```python
from build123d import *

# Parameters (mm, degrees)
SKETCH1_R           = 5
SKETCH1_R_2         = 1.5
BOSS_EXTRUDE1_DEPTH = 5
BOSS_EXTRUDE4_DEPTH = 10
FILLET5_R           = 3
FILLET7_R           = 8
CUT_EXTRUDE6_DEPTH  = 10
FILLET9_R           = 1
FILLET11_R          = 0.1


with BuildPart() as part:
    # Sketch1 → Boss-Extrude1 (new, symmetric)
    # profile 1 of 3: a face of its own
    with BuildSketch(Plane(origin=(0, 0, 0), x_dir=(0, 0, -1), z_dir=(1, 0, 0))):
        with BuildLine():
            ThreePointArc((-11, 0), (-12.464466094, -3.535533906), (-16, -5))
            Line((-16, -5), (16, -5))
            ThreePointArc((16, -5), (11, 0), (16, 5))
            Line((16, 5), (-16, 5))
            ThreePointArc((-16, 5), (-12.464466094, 3.535533906), (-11, 0))
        make_face()
    # profile 2 of 3: a face of its own
    with BuildSketch(Plane(origin=(0, 0, 0), x_dir=(0, 0, -1), z_dir=(1, 0, 0))):
        with Locations((-16, 0)):
            Circle(SKETCH1_R)
        with Locations((-16, 0)):
            Circle(SKETCH1_R_2, mode=Mode.SUBTRACT)
    # profile 3 of 3: a face of its own
    with BuildSketch(Plane(origin=(0, 0, 0), x_dir=(0, 0, -1), z_dir=(1, 0, 0))):
        with Locations((16, 0)):
            Circle(SKETCH1_R)
        with Locations((16, 0)):
            Circle(SKETCH1_R_2, mode=Mode.SUBTRACT)
    extrude(amount=BOSS_EXTRUDE1_DEPTH, both=True)

    # Sketch6 → Boss-Extrude4 (add)
    with BuildSketch(Plane(origin=(5, 0, 0), x_dir=(0, 0, -1), z_dir=(1, 0, 0))):
        with BuildLine():
            Line((20.375428035, -2.419840804), (37.626356882, 0))
            Line((37.626356882, 0), (37.626356882, -5.863506349))
            Line((37.626356882, -5.863506349), (56, -2.931753174))
            Line((56, -2.931753174), (56, -0.788607304))
            Line((56, -0.788607304), (56, 5))
            Line((56, 5), (16, 5))
            ThreePointArc((16, 5), (20.30692489, 2.539763373), (20.375428035, -2.419840804))
        make_face()
    extrude(amount=-BOSS_EXTRUDE4_DEPTH)

    # Fillet5
    fillet5_edges = [part.edges().sort_by_distance(p)[0] for p in [
        (0, 0, -37.626356882),
    ]]
    fillet(fillet5_edges, radius=FILLET5_R)

    # Fillet7
    # the kernel refuses this fillet: 8 mm, written as the material it takes off along each edge
    with BuildSketch(Plane(origin=(25, 5, -56), x_dir=(0, -1, 0), z_dir=(-1, 0, 0))) as fillet7_piece_1:
        with BuildLine():
            CenterArc((FILLET7_R, FILLET7_R), FILLET7_R, 180, 90)
            Line((0, FILLET7_R), (0, 0))
            Line((0, 0), (FILLET7_R, 0))
        make_face()
    extrude(amount=50, mode=Mode.SUBTRACT)

    # Sketch8 → Cut-Extrude6 (cut)
    with BuildSketch(Plane(origin=(5, 0, 0), x_dir=(0, 0, -1), z_dir=(1, 0, 0))):
        Polygon((56, -2.931753174), (55.020132037, -1.951885211), (54.570397118, -3.159864865), (54.024984262, -3.246892563), (53.045116299, -2.2670246), (52.59538138, -3.475004253), (52.049968524, -3.562031952), (51.070100561, -2.582163988), (50.620365642, -3.790143642), (50.074952786, -3.87717134), (49.095084823, -2.897303377), (48.645349904, -4.10528303), (48.099937048, -4.192310729), (47.120069084, -3.212442766), (46.670334166, -4.420422419), (46.12492131, -4.507450118), (45.145053346, -3.527582154), (44.695318427, -4.735561808), (44.149905571, -4.822589506), (43.170037608, -3.842721543), (42.720302689, -5.050701196), (42.174889833, -5.137728895), (41.19502187, -4.157860932), (40.745286951, -5.365840585), (40.199874095, -5.452868283), (39.220006132, -4.47300032), (38.770271213, -5.680979974), (37.626356882, -5.863506349), (46.12492131, -12.960580579), align=None)
    extrude(amount=-CUT_EXTRUDE6_DEPTH, mode=Mode.SUBTRACT)

    # Fillet9
    # the kernel refuses this fillet: 1 mm, written as the material it takes off along each edge
    with BuildSketch(Plane(origin=(7.930532836, -5.863506349, -37.626356882), x_dir=(0, 0.15756969432487367, -0.9875078690473135), z_dir=(-1, 0, 0))) as fillet9_piece_1:
        with BuildLine():
            CenterArc((FILLET9_R * 1.1722131343, -FILLET9_R), FILLET9_R, 90, 99.065860636)
            Line((FILLET9_R * 0.184705265256, -FILLET9_R * 1.15756969432), (0, 0))
            Line((0, 0), (FILLET9_R * 1.1722131343, 0))
        make_face()
    extrude(amount=15.861065672, mode=Mode.SUBTRACT)

    # Fillet11
    fillet11_edges = [part.edges().sort_by_distance(p)[0] for p in [
        (0, -2.931459557, -55.999706383),
    ]]
    fillet(fillet11_edges, radius=FILLET11_R)


solid = part.part
```
Can you work these out from the model? Positions are in its coordinate system, mm. A direction names the side the tool comes from. Coordinates: 2 decimals unless noted, no trailing zeros. Order: outer loops, then holes, each group sorted by start corner. A loop starts at its lowest first (then second) coordinate and runs counter-clockwise, first axis right, second up.
1. Thinking about a two-plate mould opening in Z: for faces 1 (the face through (0, 0, 21)), 2 (the face through (0.07, -2.547, -54.798)), 3 (the face through (0, -5, 0)), which applies, +Z half, -Z half, draft (parallel to the pull), parting line (faces both ways), or undercut?
2. If we section it at C-C (y = 3): Please give me the cut outline in (x, z).
3. For faces 4 (the face through (0, 5, -16)), 5 (the face through (0.07, -1.463, -27.196)), which set-ups out of +Z, -Z, +X, -X, +Y, -Y let a thin tool reach every point of the face, with its end or its side?
4. If we section it at B-B (z = 10): Please give me the cut outline in (x, y), then the cut area to 3 significant figures.
5. I'm going to push flat-ended pins straight in: pin 1 (3 mm diameter, centred on x = 3, y = -1.5, fed in from -Z); pin 2 (2 mm diameter, centred on x = -0.5, z = -28.5, fed in from -Y); pin 3 (1.8 mm diameter, centred on y = 0, z = -16, fed in from +X); pin 4 (1 mm diameter, centred on x = 3, y = -1.5, fed in from +Z). Where does each tip first touch, or does it pass through?
6. If we section it at A-A (x = -3.25): Give the number of separate pieces and of enclosed holes in the cut face, then the cut area to 3 significant figures.
7. I need wall thicknesses on line 1 (Y direction, x = 0, z = 16); line 2 (Z direction, x = -2, y = 0.5); line 3 (Y direction, x = -4.25, z = -45.5). Which ranges of each line are inside material? Lowest first, please.
Entries:
1. face 1: +Z half
1. face 2: undercut
1. face 3: draft
2. outline: (-5, -53.29) - (5, -53.29) - (5, 20) - (-5, 20) - close
3. face 4: +Z, -Z, +X, -X, +Y
3. face 5: +X, -X, -Y
4. outline: (-5, -5) - (5, -5) - (5, 5) - (-5, 5) - close
4. area: 100 mm2
5. pin 1: stops at z = -55.99
5. pin 2: stops at y = -1.42
5. pin 3: passes through
5. pin 4: stops at z = 20.9
6. separate pieces: 1
6. enclosed holes: 2
6. area: 647 mm2
7. line 1: y = -5 to -1.5, 1.5 to 5
7. line 2: z = -55.19 to -17.41, -14.59 to 14.59, 17.41 to 20.97
7. line 3: y = -3.88 to 5
